Design review of the part built by this model. Coordinates are the model's own, in mm. Coordinates: 2 decimals unless noted, no trailing zeros. Loops run counter-clockwise (first coordinate to the right, second up) from the corner with the lowest first, then second, coordinate; pieces in that order, holes last. Notation, with made-up numbers: (43.5, 63.5) -> (95.5, 63.5) arc R16 ccw to (95.5, 93.5) -> close; hole circle Ø11 at (59.25, 5). An arc over 180 degrees is marked (long way). One line per item, written item: value. Start each with the question number.
1. Add section A-A on x = 0. Write out the cut boundary in (y, z).
2. Add section D-D on x = 3.5. Write out the cut boundary in (y, z), plus the area to 3 significant figures.
3. Insertion check: pin 1 (1.2 mm diameter, centred on x = 0, y = 0, fed in from -Z); pin 2 (1.5 mm diameter, centred on x = 4.5, z = 1, fed in from -Y); pin 3 (2 mm diameter, centred on x = 8.5, z = 4, fed in from -Y); pin 4 (1.5 mm diameter, centred on y = 4.5, z = 1.5, fed in from -X). Each pin has a flat end and moves straight along its axis. Give the tip position at first contact, or say it passes through.
4. Add section B-B on z = 1.25. Write out the cut boundary in (x, y), plus the area to 3 significant figures.
5. Draft analysis for pull direction Y (two halves, no side actions). For faces 1 (the flat face through (8, 0, 3)), 2 (the flat face through (2, 5, 6)), 3 (the cylindrical face through (4.873, 8.733, 2.958)), 4 (the cylindrical face through (0, 1, 3)), state which applies: pulls with the +Y half, pulls with the -Y half, needs draft (parallel to the pull), parting line crosses it, or undercut.
6. Add section C-C on y = -1.25. Write out the cut boundary in (x, z), plus the area to 3 significant figures.
7. For probe 1 along Y at (x, z) = (0, 1.3); probe 2 along X at (y, z) = (-0.75, 0.6); probe 3 along X at (y, z) = (0.5, 4.95), list the stretches that pass through material, from the lowest coordinate up.
Autodesk Fusion 360 part; units mm, degrees
sketch "Sketch1" plane through (0, 0, 0) normal (0, 0, 1) x (1, 0, 0) in component "Component"
  circle A0 centre (0, 0) radius 1
  circle A1 centre (0, 0) radius 2.5
  line L0 (0, 0) -> (10, 0) construction
  line L1 (0, 0) -> (-5, 8.6603) construction
  line L2 (0, 0) -> (7.8295, 0) construction
  arc A2 (10, 0) -> (-5, 8.6603) centre (0, 0) ccw
  line L3 (-5, 8.6603) -> (-1.25, 2.1651)
  line L4 (2.5, 0) -> (10, 0)
  line L5 (-1.25, 2.1651) -> (-2.75, 4.7631) construction
  arc A3 (-2.3654, 0.8093) -> (-2.75, 4.7631) centre (-6.9069, 2.3631) ccw
  line L6 (2.5, 0) -> (5.5, 0)
  arc A4 (5.5, 0) -> (1.8836, -1.6438) centre (5.5, -4.8) ccw
  dimension "d1" = 2
  dimension "d2" = 5
  dimension "d3" = 10
  dimension "d4" = 120
  dimension "d5" = 10
  dimension "d6" = 3
  dimension "d7" = 3
extrude "Extrude1" add sketch "Sketch1" along normal blind 6 in component "Component"
component "Component" placed x (1, 0, 0) y (0, 1, 0) z (0, 0, 1) at (0, 0, 0)
equation "d5 = d3"
Worked answers:
1. outline: (-2.5, 0) -> (-1, 0) -> (-1, 6) -> (-2.5, 6) -> close; (1, 0) -> (10, 0) -> (10, 6) -> (1, 6) -> close
2. outline: (-0.44, 0) -> (9.37, 0) -> (9.37, 6) -> (-0.44, 6) -> close
2. area: 58.8 mm²
3. pin 1: passes through
3. pin 2: stops at y = -0.33
3. pin 3: stops at y = 0
3. pin 4: stops at x = -3.03
4. outline: (-5, 8.66) -> (-2.75, 4.76) arc R4.8 cw to (-2.37, 0.81) arc R2.5 ccw to (1.88, -1.64) arc R4.8 cw to (5.5, 0) -> (10, 0) arc R10 ccw to start; hole circle Ø2 at (0, 0)
4. area: 117 mm²
5. face 1: pulls with the -Y half
5. face 2: needs draft
5. face 3: pulls with the +Y half
5. face 4: undercut
6. outline: (-2.17, 0) -> (2.27, 0) -> (2.27, 6) -> (-2.17, 6) -> close
6. area: 26.6 mm²
7. probe 1: y = -2.5 to -1, 1 to 10
7. probe 2: x = -2.38 to -0.66, 0.66 to 2.92
7. probe 3: x = -2.45 to -0.87, 0.87 to 9.99
